Geometry check sheet. Reference: the model listing, model coordinates, mm. Face numbers are marked on the shaded views. A direction names the side the tool comes from. Give positions to 0.01 mm unless a question says otherwise; leave off trailing zeros. Order: outer loops, then holes, each group sorted by start corner. A loop starts at its lowest first (then second) coordinate and runs counter-clockwise, first axis right, second up. Notation, with made-up numbers: M 77,38 L 133,38 A11 cw 133,47 Z; hole C 39.25,68.25 d5. An arc over 180 degrees is marked long. Answer as CSV lines item,"result".
from build123d import *

# Parameters (mm, degrees)
F2_R     = 5.125
F3_DEPTH = 5.25
F4_W     = 5.5
F4_H     = 2
F5_DEPTH = 7.5


with BuildPart() as f1:
    # F0 (on Front) → F1 (revolve)
    with BuildSketch(Plane.XZ):
        with BuildLine():
            Line((0, 8.5), (0, 0))
            Line((0, 0), (7, 0))
            Line((7, 0), (7, 5.5))
            ThreePointArc((7, 5.5), (6.12132, 7.62132), (4, 8.5))
            Line((4, 8.5), (0, 8.5))
        make_face()
    revolve(axis=Axis((0, 0, 2.545049), (0, 0, 1)))

    # F2 (on face) → F3 (cut)
    with BuildSketch(Plane(origin=(0, 0, 0), x_dir=(1, 0, 0), z_dir=(0, 0, -1))):
        Circle(F2_R)
    extrude(amount=-F3_DEPTH, mode=Mode.SUBTRACT)

    # F4 (on Front) → F5 (cut, symmetric)
    with BuildSketch(Plane.XZ):
        with Locations((0, 6.25)):
            Rectangle(F4_W, F4_H)
    extrude(amount=F5_DEPTH, both=True, mode=Mode.SUBTRACT)


solid = f1.part
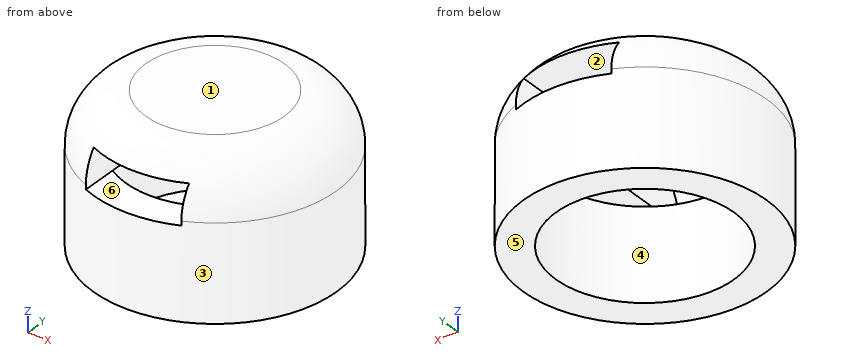
(1) Material ranges on line 1 (Y direction, x = -3, z = 3); line 2 (Y direction, x = 0, z = 3.8) (3 decimals); line 3 (Z direction, x = 1, y = -5.5), recorded low to high.
The answers:
line 1,"y = -6.32 to -4.16, 4.16 to 6.32"
line 2,"y = -7 to -5.125, 5.125 to 7"
line 3,"z = 0 to 5.25, 7.25 to 8.04"
(2) Draft check along X on the marked faces 1, 2 and 3. Enter one of: +X half, -X half, draft (parallel to the pull), parting line (faces both ways), or undercut.
The answers:
face 1,"draft"
face 2,"undercut"
face 3,"parting line"
(3) Gauge pin test, flat ends, axial feed: P1, Ø3, axis at x = 0, y = 1.5, coming from the -Z side; P2, Ø1, axis at y = -3, z = 2, coming from the +X side; P3, Ø1.5, axis at x = 3, z = 3.5, coming from the +Y side. Record the tip position at first contact, or that the pin passes through.
The answers:
P1,"stops at z = 7.25"
P2,"stops at x = 6.54"
P3,"stops at y = 6.63"
(4) Section check C-C on z = 6.5. Enter the section's corners in (x, y), then the cut area to 3 significant figures.
The answers:
outline,"M -2.75,-6.25 L -2.75,6.25 A6.83 ccw Z; M 2.75,-6.25 A6.83 ccw 2.75,6.25 Z"
area,"73.5 mm2"
(5) Section check D-D on z = 2. Enter the section's corners in (x, y) (3 decimals), then the cut area to 3 significant figures.
The answers:
outline,"C 0,0 d14; hole C 0,0 d10.25"
area,"71.4 mm2"
(6) Section check A-A on x = 0. Enter the section's corners in (y, z) (3 decimals), then the cut area to 3 significant figures.
The answers:
outline,"M -7,0 L -5.125,0 L -5.125,5.25 L -7,5.25 Z; M -6.437,7.25 L 6.437,7.25 A3 ccw 4,8.5 L -4,8.5 A3 ccw Z; M 5.125,0 L 7,0 L 7,5.25 L 5.125,5.25 Z"
area,"34.0 mm2"
(7) Section check B-B on y = 0. Enter the section's corners in (x, z) (3 decimals), then the cut area to 3 significant figures.
The answers:
outline,"M -7,0 L -5.125,0 L -5.125,5.25 L -2.75,5.25 L -2.75,7.25 L 2.75,7.25 L 2.75,5.25 L 5.125,5.25 L 5.125,0 L 7,0 L 7,5.5 A3 ccw 4,8.5 L -4,8.5 A3 ccw -7,5.5 Z"
area,"50.3 mm2"
(8) Tool access check on the marked faces 4, 5 and 6. Record the directions out of +Z, -Z, +X, -X, +Y, -Y that give a thin tool (end or side, any length) a straight path to the whole face; none if there is none.
The answers:
face 4,"-Z"
face 5,"-Z, +X, -X, +Y, -Y"
face 6,"+Y, -Y"
